Source: CAD feature listing. Evaluate the final solid. Frame: model axes, mm. A direction names the side the tool comes from. Coordinates: 2 decimals unless noted, no trailing zeros. Order: outer loops, then holes, each group sorted by start corner. A loop starts at its lowest first (then second) coordinate and runs counter-clockwise, first axis right, second up.
```python
from build123d import *

# Parameters (mm, degrees)
MOUNTING_FLANGE_START                          = -4
SKETCH1_R                                      = 11
MOUNTING_FLANGE_DEPTH                          = 4
SKETCH2_R                                      = 2.75
D5P5_CENTRAL_POST_DEPTH                        = 32.81
CLOSED_FLOOR_BELOW_SHAFT_NOSE_START            = 32.8
SKETCH3_R                                      = 10
CLOSED_FLOOR_BELOW_SHAFT_NOSE_DEPTH            = 2.2
SHAFT_AND_CLIP_CLEARANCE_START                 = 35
SKETCH4_R                                      = 10
SKETCH4_R_2                                    = 5.7
SHAFT_AND_CLIP_CLEARANCE_DEPTH                 = 6.5
LOWER_686ZZ_SEAT_START                         = 41.5
SKETCH5_R                                      = 10
SKETCH5_R_2                                    = 6.5
LOWER_686ZZ_SEAT_DEPTH                         = 5
SKETCH6_R                                      = 1
BASE_THREE_M2_BLIND_THREAD_MAJOR_ENVELOP_DEPTH = 3.6
TOP_CAP_THREE_M2_BLIND_THREAD_MAJOR_ENVE_START = -4.3
SKETCH7_R                                      = 1
TOP_CAP_THREE_M2_BLIND_THREAD_MAJOR_ENVE_DEPTH = 4.3


with BuildPart() as part:
    # Sketch1 → Mounting_Flange (new body)
    with BuildSketch(Plane.XY.offset(MOUNTING_FLANGE_START)):
        Circle(SKETCH1_R)
    extrude(amount=MOUNTING_FLANGE_DEPTH)

    # Sketch2 → D5p5_Central_Post (add)
    with BuildSketch(Plane.XY):
        Circle(SKETCH2_R)
    extrude(amount=D5P5_CENTRAL_POST_DEPTH)

    # Sketch3 → Closed_Floor_Below_Shaft_Nose (add)
    with BuildSketch(Plane.XY.offset(CLOSED_FLOOR_BELOW_SHAFT_NOSE_START)):
        Circle(SKETCH3_R)
    extrude(amount=CLOSED_FLOOR_BELOW_SHAFT_NOSE_DEPTH)

    # Sketch4 → Shaft_And_Clip_Clearance (add)
    with BuildSketch(Plane.XY.offset(SHAFT_AND_CLIP_CLEARANCE_START)):
        Circle(SKETCH4_R)
        with Locations(Location((0, 0, 0), (0, 0, 180))):
            Circle(SKETCH4_R_2, mode=Mode.SUBTRACT)
    extrude(amount=SHAFT_AND_CLIP_CLEARANCE_DEPTH)

    # Sketch5 → Lower_686ZZ_Seat (add)
    with BuildSketch(Plane.XY.offset(LOWER_686ZZ_SEAT_START)):
        Circle(SKETCH5_R)
        Circle(SKETCH5_R_2, mode=Mode.SUBTRACT)
    extrude(amount=LOWER_686ZZ_SEAT_DEPTH)

    # Sketch6 → Base_Three_M2_Blind_Thread_Major_Envelopes (cut)
    with BuildSketch(Plane(origin=(0, 0, -4), x_dir=(-1, 0, 0), z_dir=(0, 0, -1))):
        with Locations((-7.188010851, 4.15)):
            Circle(SKETCH6_R)
        with Locations((7.188010851, 4.15)):
            Circle(SKETCH6_R)
        with Locations((0, -8.3)):
            Circle(SKETCH6_R)
    extrude(amount=-BASE_THREE_M2_BLIND_THREAD_MAJOR_ENVELOP_DEPTH, mode=Mode.SUBTRACT)

    # Sketch7 → Top_Cap_Three_M2_Blind_Thread_Major_Envelopes (cut)
    with BuildSketch(Plane.XY.offset(46.5).offset(TOP_CAP_THREE_M2_BLIND_THREAD_MAJOR_ENVE_START)):
        with Locations(Location((7.188010851, 4.15, 0), (0, 0, 180))):
            Circle(SKETCH7_R)
        with Locations(Location((-7.188010851, 4.15, 0), (0, 0, 180))):
            Circle(SKETCH7_R)
        with Locations(Location((0, -8.3, 0), (0, 0, 180))):
            Circle(SKETCH7_R)
    extrude(amount=TOP_CAP_THREE_M2_BLIND_THREAD_MAJOR_ENVE_DEPTH, mode=Mode.SUBTRACT)


solid = part.part
```
1. Section query A-A on x = -3.25. Return loops of the section in (y, z).
Findings:
outline: (-10.51, -4) - (10.51, -4) - (10.51, 0) - (-10.51, 0) - close; (-9.46, 32.8) - (9.46, 32.8) - (9.46, 46.5) - (5.63, 46.5) - (5.63, 41.5) - (4.68, 41.5) - (4.68, 35) - (-4.68, 35) - (-4.68, 41.5) - (-5.63, 41.5) - (-5.63, 46.5) - (-9.46, 46.5) - close
2. Section query C-C on z = 38.5. Return loops of the section in (x, y).
Findings:
outline: circle Ø20 at (0, 0); hole circle Ø11.4 at (0, 0)
3. Access query for faces 5 (the face through (-2.38, -10.74, -2.03)), 6 (the face through (0, -6, 41.5)), 7 (the face through (2.1, -2.1, 32.8)), 8 (the face through (0.13, -7.31, -2.23)). Directions: +Z, -Z, +X, -X, +Y, -Y. A direction counts if a zero-diameter tool reaches every point of the face in a straight line with its end or side. Return the directions, or none.
Findings:
face 5: +Z, -Z
face 6: +Z
face 7: none
face 8: -Z
4. Draft query along Y for faces 1 (the face through (6.264, 3.767, -2.225)), 2 (the face through (6.264, 4.533, 44.32)), 3 (the face through (0, 0, -4)), 4 (the face through (-2.17, -9.76, 39.55)). Return one class per face: released by +Y, released by -Y, zero draft, split by the parting line, or undercut.
Findings:
face 1: undercut
face 2: undercut
face 3: zero draft
face 4: split by the parting line
5. Ray query, line 1 (Z direction, x = -1, y = -3.75); line 2 (Y direction, x = 0, z = -3.15); line 3 (Z direction, x = -5, y = -4.25). Return the intervals inside material, ascending.
Findings:
line 1: z = -4 to 0, 32.8 to 35
line 2: y = -11 to -9.3, -7.3 to 11
line 3: z = -4 to 0, 32.8 to 46.5
6. Pin query (flat end, axial travel): P1, Ø1, axis at x = -7.5, y = 4, coming from the -Z side; P2, Ø6, axis at x = 4.5, z = 4.5, coming from the +Y side; P3, Ø2, axis at x = -0.5, z = 35.5, coming from the +Y side. Return the tip coordinate at first contact, or that it passes through.
Findings:
P1: stops at z = -0.4
P2: stops at y = 2.3
P3: stops at y = 10
7. Section query B-B on y = -8.3. Return loops of the section in (x, z).
Findings:
outline: (-7.22, -4) - (-1, -4) - (-1, -0.4) - (1, -0.4) - (1, -4) - (7.22, -4) - (7.22, 0) - (-7.22, 0) - close; (-5.58, 32.8) - (5.58, 32.8) - (5.58, 46.5) - (1, 46.5) - (1, 42.2) - (-1, 42.2) - (-1, 46.5) - (-5.58, 46.5) - close
8. Section query D-D on y = 0. Return loops of the section in (x, z).
Findings:
outline: (-11, -4) - (11, -4) - (11, 0) - (2.75, 0) - (2.75, 32.8) - (10, 32.8) - (10, 46.5) - (6.5, 46.5) - (6.5, 41.5) - (5.7, 41.5) - (5.7, 35) - (-5.7, 35) - (-5.7, 41.5) - (-6.5, 41.5) - (-6.5, 46.5) - (-10, 46.5) - (-10, 32.8) - (-2.75, 32.8) - (-2.75, 0) - (-11, 0) - close
